For this review, take the finished solid that the model builds, in its own axes (mm). A direction names the side the tool comes from. Round coordinates to 2 decimals unless told otherwise and drop trailing zeros. Order: outer loops, then holes, each group sorted by start corner. A loop starts at its lowest first (then second) coordinate and runs counter-clockwise, first axis right, second up. Notation, with made-up numbers: (1, -9.5) - (7, -9.5) arc R17 ccw to (7, -5.5) - close; hole circle Ø4 at (4.25, 89.5). An arc over 180 degrees is marked (long way). One line per item, written item: value.
```python
from build123d import *

# Parameters (mm, degrees)
SKETCH1_R             = 95
SKETCH1_R_2           = 1.5
SKETCH1_R_3           = 2
SKETCH1_R_4           = 3.5
BOSS_EXTRUDE1_DEPTH   = 5
BODY_MOVE_COPY1_ANGLE = 90


with BuildPart() as part:
    # Sketch1 → Boss-Extrude1 (new body)
    with BuildSketch(Plane(origin=(0, 0, 0), x_dir=(1, 0, 0), z_dir=(0, 1, 0))):
        Circle(SKETCH1_R)
        with Locations((48.790367902, 48.790367902)):
            Circle(SKETCH1_R_2, mode=Mode.SUBTRACT)
        with Locations((0, 40)):
            Circle(SKETCH1_R_3, mode=Mode.SUBTRACT)
        with Locations((40, 0)):
            Circle(SKETCH1_R_3, mode=Mode.SUBTRACT)
        with Locations((0, -40)):
            Circle(SKETCH1_R_3, mode=Mode.SUBTRACT)
        with Locations((-40, 0)):
            Circle(SKETCH1_R_3, mode=Mode.SUBTRACT)
        with Locations((48.790367902, -48.790367902)):
            Circle(SKETCH1_R_2, mode=Mode.SUBTRACT)
        with Locations((-48.790367902, -48.790367902)):
            Circle(SKETCH1_R_2, mode=Mode.SUBTRACT)
        with Locations((-48.790367902, 48.790367902)):
            Circle(SKETCH1_R_2, mode=Mode.SUBTRACT)
        with Locations((80, 0)):
            Circle(SKETCH1_R_4, mode=Mode.SUBTRACT)
        with Locations((69.282032303, -40)):
            Circle(SKETCH1_R_4, mode=Mode.SUBTRACT)
        with Locations((40, -69.282032303)):
            Circle(SKETCH1_R_4, mode=Mode.SUBTRACT)
        with Locations((0, -80)):
            Circle(SKETCH1_R_4, mode=Mode.SUBTRACT)
        with Locations((-40, -69.282032303)):
            Circle(SKETCH1_R_4, mode=Mode.SUBTRACT)
        with Locations((-69.282032303, -40)):
            Circle(SKETCH1_R_4, mode=Mode.SUBTRACT)
        with Locations((-80, 0)):
            Circle(SKETCH1_R_4, mode=Mode.SUBTRACT)
        with Locations((-69.282032303, 40)):
            Circle(SKETCH1_R_4, mode=Mode.SUBTRACT)
        with Locations((-40, 69.282032303)):
            Circle(SKETCH1_R_4, mode=Mode.SUBTRACT)
        with Locations((0, 80)):
            Circle(SKETCH1_R_4, mode=Mode.SUBTRACT)
        with Locations((40, 69.282032303)):
            Circle(SKETCH1_R_4, mode=Mode.SUBTRACT)
        with Locations((69.282032303, 40)):
            Circle(SKETCH1_R_4, mode=Mode.SUBTRACT)
        with BuildLine():
            Line((10, -21), (10, -30.000108076))
            ThreePointArc((10, -30.000108076), (9.414180319, -31.414301502), (7.999957489, -32.000050194))
            Line((7.999957489, -32.000050194), (-8.000158272, -32.000050194))
            ThreePointArc((-8.000158272, -32.000050194), (-9.414280711, -31.414259919), (-10, -30.000108076))
            Line((-10, -30.000108076), (-10, -21))
            Line((-10, -21), (-16.005742178, -21))
            ThreePointArc((-16.005742178, -21), (-19.538404995, -19.534344662), (-21, -16))
            Line((-21, -16), (-21, 16))
            ThreePointArc((-21, 16), (-19.535533906, 19.535533906), (-16, 21))
            Line((-16, 21), (16, 21))
            ThreePointArc((16, 21), (19.535388079, 19.536388365), (21.000355251, 16.001561768))
            Line((21.000355251, 16.001561768), (21.000355251, -16.001561768))
            ThreePointArc((21.000355251, -16.001561768), (19.536346588, -19.535991337), (16.001917019, -21))
            Line((16.001917019, -21), (10, -21))
        make_face(mode=Mode.SUBTRACT)
    extrude(amount=BOSS_EXTRUDE1_DEPTH)


with BuildPart() as part_1:
    # Body-Move/Copy1: moved
    add(part.part.rotate(Axis((0, 2.5, 0), (1, 0, 0)), BODY_MOVE_COPY1_ANGLE))


solid = part_1.part
```
Item 1: Take a section at A-A (x = -80). Write out the cut boundary in (y, z).
Returned:
outline: (-48.73, -2.5) - (-1, -2.5) - (-1, 2.5) - (-48.73, 2.5) - close; (6, -2.5) - (53.73, -2.5) - (53.73, 2.5) - (6, 2.5) - close
Item 2: The part is to be moulded in two halves that separate along X. For faces 3 (the cylindrical face through (19.496, 22.075, -0.035)), 4 (the cylindrical face through (90.61, 31.04, -0.04)), 5 (the flat face through (-1, 25, -2.5)), say which applies: +X half, -X half, draft (parallel to the pull), parting line (faces both ways), or undercut.
Returned:
face 3: undercut
face 4: parting line
face 5: draft
Item 3: Machinability: for faces 1 (the flat face through (-1, 25, 2.5)), 2 (the flat face through (0, -29.5, 0)), which of the approach directions +Z, -Z, +X, -X, +Y, -Y give a long, thin tool a straight path to every point of the face, cutting with its end or side? Answer none if there is none.
Returned:
face 1: +Z, +X, -X, +Y, -Y
face 2: +Z, -Z
Item 4: Take a section at B-B (y = -6.5). Write out the cut boundary in (x, z), plus the area to 3 significant figures.
Returned:
outline: (-94.57, -2.5) - (-21, -2.5) - (-21, 2.5) - (-94.57, 2.5) - close; (21, -2.5) - (94.57, -2.5) - (94.57, 2.5) - (21, 2.5) - close
area: 736 mm^2
Item 5: Take a section at D-D (z = 1.15). Count the separate pieces of the cut face and the enclosed holes in it, plus the area to 3 significant figures.
Returned:
separate pieces: 1
enclosed holes: 21
area: 25,900 mm^2
Item 6: For P1, Ø2.5, axis at x = 48.79, y = -46.29, coming from the +Z side; P2, Ø3, axis at x = -60.5, z = 1.5, coming from the +Y side; P3, Ø2.5, axis at y = -24, z = 0.5, coming from the -X side; P4, Ø3, axis at x = 47.5, z = -2, coming from the -Y side, all flat-tipped, find the tip position at first contact; note any pin that passes through.
Returned:
P1: through
P2: y = 76.96
P3: x = -91.58
P4: y = -80.62
Item 7: Take a section at C-C (y = 31.5). Write out the cut boundary in (x, z).
Returned:
outline: (-90.47, -2.5) - (90.47, -2.5) - (90.47, 2.5) - (-90.47, 2.5) - close
Item 8: Wall thickness on line 1 (Y direction, x = 0, z = -1.35); line 2 (Y direction, x = -40, z = 0.55); line 3 (X direction, y = 5, z = -0.05): over which ranges is each line inside the solid? List them lowest first.
Returned:
line 1: -92.5 to -81, -74 to -39.5, -35.5 to -29.5, 23.5 to 40.5, 44.5 to 79, 86 to 97.5
line 2: -83.67 to -70.28, -63.28 to 0.5, 4.5 to 68.28, 75.28 to 88.67
line 3: -94.97 to -82.45, -77.55 to -21, 21 to 77.55, 82.45 to 94.97
